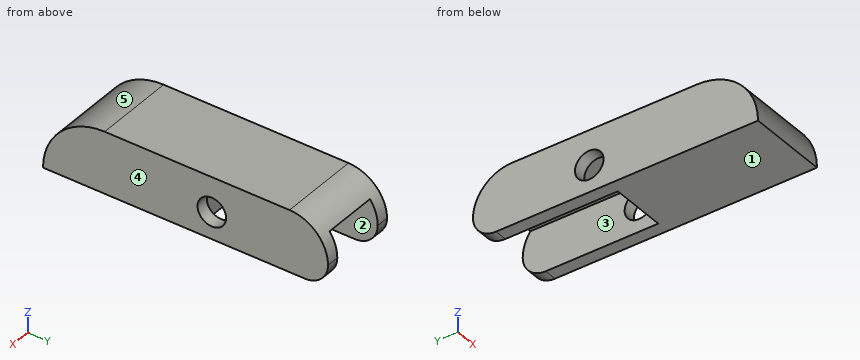
from build123d import *

# Parameters (mm, degrees)
SKETCH1_W               = 13.335
SKETCH1_H               = 46.99
BOSS_EXTRUDE1_DEPTH     = 10.16
FILLET5_R               = 3.81
SKETCH2_W               = 9.144
SKETCH2_H               = 22.352
CUT_EXTRUDE1_DEPTH      = 7.62
CUT_EXTRUDE2_DEPTH      = 50.890960354
CUT_EXTRUDE2_DEPTH_BACK = 50.890960354
SKETCH3_R               = 2.35585
FILLET4_R               = 6.35
FILLET6_R               = 10.16


# Some blends are built 0.0001 mm under size
with BuildPart() as part:
    # Sketch1 → Boss-Extrude1 (new body)
    with BuildSketch(Plane.XY):
        with Locations((6.6675, 23.495)):
            Rectangle(SKETCH1_W, SKETCH1_H)
    extrude(amount=BOSS_EXTRUDE1_DEPTH)

    # Fillet5
    fillet5_edges = [part.edges().sort_by_distance(p)[0] for p in [
        (6.6675, 46.99, 0),
    ]]
    fillet(fillet5_edges, radius=FILLET5_R)

    # Sketch2 → Cut-Extrude1 (cut)
    with BuildSketch(Plane(origin=(0, 0, 0), x_dir=(-1, 0, 0), z_dir=(0, 0, -1))):
        with Locations((-6.6675, 35.814)):
            Rectangle(SKETCH2_W, SKETCH2_H)
    extrude(amount=-CUT_EXTRUDE1_DEPTH, mode=Mode.SUBTRACT)

    # Sketch3 → Cut-Extrude2 (cut, two sides: drawn at the far end of the back side and taken through both)
    with BuildSketch(Plane.ZY.offset(-CUT_EXTRUDE2_DEPTH_BACK)):
        with Locations((4.4323, 27.8257)):
            Circle(SKETCH3_R)
    extrude(amount=CUT_EXTRUDE2_DEPTH + CUT_EXTRUDE2_DEPTH_BACK, mode=Mode.SUBTRACT)

    # Fillet4
    # the kernel refuses this fillet: 6.35 mm, written as the material it takes off along each edge
    with BuildSketch(Plane(origin=(29.21, 46.99, 10.16), x_dir=(0, 0, -1), z_dir=(-1, 0, 0))) as fillet4_piece_1:
        with BuildLine():
            CenterArc((FILLET4_R, FILLET4_R), FILLET4_R, 180, 90)
            Line((0, FILLET4_R), (0, 0))
            Line((0, 0), (FILLET4_R, 0))
        make_face()
    extrude(amount=45.085, mode=Mode.SUBTRACT)

    # Fillet6
    fillet6_edges = [part.edges().sort_by_distance(p)[0] for p in [
        (6.6675, 0, 10.16),
    ]]
    fillet(fillet6_edges, radius=FILLET6_R - 0.0001)  # a hair under: the kernel refuses the full size


solid = part.part
Build history of the part. All positions in model axes, mm. Face numbers are marked on the shaded views. A direction names the side the tool comes from. Round coordinates to 2 decimals unless told otherwise and drop trailing zeros. Loops run counter-clockwise (first coordinate to the right, second up) from the corner with the lowest first, then second, coordinate; pieces in that order, holes last. Notation, with made-up numbers: (22.5, 4.5) -> (46.5, 4.5) arc R19 ccw to (46.5, 8.5) -> close; hole circle Ø6 at (79.5, 52). An arc over 180 degrees is marked (long way). One line per item, written item: value. Start each with the question number.
Q1. Cut at C-C on z = 5.5. List the corners of the cut face in (x, y) (1 decimal).
Q2. Drop a flat-ended pin along its axis: pin 1 Ø2.5 at (x, y) = (4.5, 39) entering from -Z. Give the stop position or say it passes through.
Q3. Probe line 1 along X through (y, z) = (33, 1.25) (1 decimal); line 2 along Z through (x, y) = (0.5, 10); line 3 along Y through (x, z) = (12, 4). List the from-to ranges inside material, lowest first.
Q4. 3-axis set-ups, long thin cutter, end or side, ignore diameter. For the marked faces 1 and 2: which of +Z, -Z, +X, -X, +Y, -Y reach the whole face in a straight line?
Q5. Two-plate mould, pull along X, no slides. Class the marked faces 3, 4 and 5: released by +X, released by -X, zero draft, split by the parting line, or undercut.
Q6. Cut at B-B on y = 26. List the corners of the cut face in (x, z) (1 decimal), plus the area to 3 significant figures.
Computed:
1. outline: (0, 1.6) -> (13.3, 1.6) -> (13.3, 25.7) -> (11.2, 25.7) -> (11.2, 24.6) -> (2.1, 24.6) -> (2.1, 25.7) -> (0, 25.7) -> close; (0, 29.9) -> (2.1, 29.9) -> (2.1, 46.8) -> (0, 46.8) -> close; (11.2, 29.9) -> (13.3, 29.9) -> (13.3, 46.8) -> (11.2, 46.8) -> close
2. pin 1: z = 7.62
3. line 1: 0 to 2.1, 11.2 to 13.3
3. line 2: 0 to 10.16
3. line 3: 0.82 to 25.51, 30.14 to 46.99
4. face 1: -Z, +X, -X, +Y, -Y
4. face 2: -Z, +Y
5. face 3: undercut
5. face 4: released by +X
5. face 5: zero draft
6. outline: (0, 0) -> (2.1, 0) -> (2.1, 2.9) -> (0, 2.9) -> close; (0, 5.9) -> (2.1, 5.9) -> (2.1, 7.6) -> (11.2, 7.6) -> (11.2, 5.9) -> (13.3, 5.9) -> (13.3, 10.2) -> (0, 10.2) -> close; (11.2, 0) -> (13.3, 0) -> (13.3, 2.9) -> (11.2, 2.9) -> close
6. area: 53.3 mm²
